Design review of the part built by this model. Coordinates are the model's own, in mm. Face numbers are marked on the shaded views. Give positions to 0.01 mm unless a question says otherwise; leave off trailing zeros. Write each loop counter-clockwise with the first axis right and the second up, starting at its lowest first coordinate (ties: lowest second). Pieces come first, ordered by that corner, then holes. Notation, with made-up numbers: M -28.5,66.25 L -24.5,66.25 A13 ccw -24.5,91.25 Z; hole C 60.25,37 d1. An arc over 180 degrees is marked long. Answer in a Markdown table with one row per item.
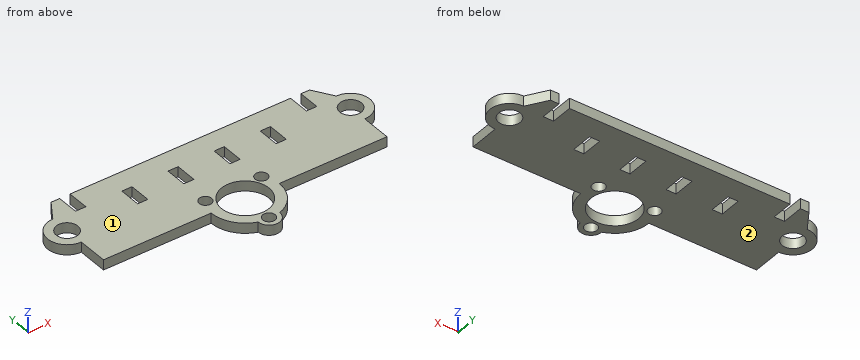
```python
from build123d import *

# Parameters (mm, degrees)
SKETCH2_R           = 7
SKETCH2_R_2         = 3.175
SKETCH2_R_3         = 1.8161
BOSS_EXTRUDE1_DEPTH = 2.9972
SKETCH3_W           = 2.9972
SKETCH3_H           = 6.35
CUT_EXTRUDE1_DEPTH  = 55.254506352


with BuildPart() as part:
    # Sketch2 → Boss-Extrude1 (new body)
    with BuildSketch(Plane.XY):
        with BuildLine():
            Line((-35.56, 26.035), (-38.1, 26.035))
            Line((-38.1, 26.035), (-41.790231571, 20.32))
            ThreePointArc((-41.790231571, 20.32), (-47.505231571, 14.605), (-41.790231571, 8.89))
            Line((-41.790231571, 8.89), (-41.790231571, 0))
            Line((-41.790231571, 0), (-10.040231571, 0))
            ThreePointArc((-10.040231571, 0), (-8.145059399, -5.87062666), (-3.175, -9.525))
            ThreePointArc((-3.175, -9.525), (0, -12.7), (3.175, -9.525))
            ThreePointArc((3.175, -9.525), (8.145059399, -5.87062666), (10.040231571, 0))
            Line((10.040231571, 0), (41.790231571, 0))
            Line((41.790231571, 0), (41.790231571, 8.89))
            ThreePointArc((41.790231571, 8.89), (47.505231571, 14.605), (41.790231571, 20.32))
            Line((41.790231571, 20.32), (38.1, 26.035))
            Line((38.1, 26.035), (35.56, 26.035))
            Line((35.56, 26.035), (35.56, 19.685))
            Line((35.56, 19.685), (32.512, 19.685))
            Line((32.512, 19.685), (32.512, 26.035))
            Line((32.512, 26.035), (-32.512, 26.035))
            Line((-32.512, 26.035), (-32.512, 19.685))
            Line((-32.512, 19.685), (-35.56, 19.685))
            Line((-35.56, 19.685), (-35.56, 26.035))
        make_face()
        with Locations(Location((0, 0, 0), (0, 0, 180))):
            Circle(SKETCH2_R, mode=Mode.SUBTRACT)
        with Locations(Location((-41.790231571, 14.605, 0), (0, 0, 180))):
            Circle(SKETCH2_R_2, mode=Mode.SUBTRACT)
        with Locations(Location((-8.248891971, 4.7625, 0), (0, 0, 180))):
            Circle(SKETCH2_R_3, mode=Mode.SUBTRACT)
        with Locations(Location((0, -9.525, 0), (0, 0, 180))):
            Circle(SKETCH2_R_3, mode=Mode.SUBTRACT)
        with Locations(Location((41.790231571, 14.605, 0), (0, 0, 180))):
            Circle(SKETCH2_R_2, mode=Mode.SUBTRACT)
        with Locations(Location((8.248891971, 4.7625, 0), (0, 0, 180))):
            Circle(SKETCH2_R_3, mode=Mode.SUBTRACT)
    extrude(amount=BOSS_EXTRUDE1_DEPTH)

    # Sketch3 → Cut-Extrude1 (cut, through all)
    with BuildSketch(Plane(origin=(0, 0, 0), x_dir=(-1, 0, 0), z_dir=(0, 0, -1))):
        with Locations((-20.40636, 16.51)):
            Rectangle(SKETCH3_W, SKETCH3_H)
        with Locations((-6.80212, 16.51)):
            Rectangle(SKETCH3_W, SKETCH3_H)
        with Locations((6.80212, 16.51)):
            Rectangle(SKETCH3_W, SKETCH3_H)
        with Locations((20.40636, 16.51)):
            Rectangle(SKETCH3_W, SKETCH3_H)
    extrude(amount=-CUT_EXTRUDE1_DEPTH, mode=Mode.SUBTRACT)


solid = part.part
```
1) Add section A-A (x = 0). Write out the cut boundary in (y, z) (3 decimals), and give its area (3 significant figures).
Geometry says:
| item | result |
|---|---|
| outline | M -12.7,0 L -11.341,0 L -11.341,2.997 L -12.7,2.997 Z; M -7.709,0 L -7,0 L -7,2.997 L -7.709,2.997 Z; M 7,0 L 26.035,0 L 26.035,2.997 L 7,2.997 Z |
| area | 63.2 mm^2 |
2) The part is to be moulded in two halves that separate along Z. For the marked faces 1 and 2, say which applies: released by +Z, released by -Z, zero draft, split by the parting line, or undercut.
Geometry says:
| item | result |
|---|---|
| face 1 | released by +Z |
| face 2 | released by -Z |
3) Add section C-C (x = 40). Write out the cut boundary in (y, z), and give its area (3 significant figures).
Geometry says:
| item | result |
|---|---|
| outline | M 0,0 L 11.98,0 L 11.98,3 L 0,3 Z; M 17.23,0 L 23.09,0 L 23.09,3 L 17.23,3 Z |
| area | 53.5 mm^2 |
4) To check wall thickness, follow probe 1 along Y at (x, z) = (0, 1.1) (3 decimals); probe 2 along X at (y, z) = (21, 0.15); probe 3 along X at (y, z) = (13, 0.9). State the ranges of each line that lie inside material, in increasing order. Write a range as [from, to].
Geometry says:
| item | result |
|---|---|
| probe 1 | [-12.7, -11.341], [-7.709, -7], [7, 26.035] |
| probe 2 | [-41.35, -35.56], [-32.51, 32.51], [35.56, 41.35] |
| probe 3 | [-47.28, -44.53], [-39.05, 39.05], [44.53, 47.28] |
5) Add section D-D (z = 1.3). Count the separate pieces of the cut face and the enclosed holes in it, and give its area (3 significant figures).
Geometry says:
| item | result |
|---|---|
| separate pieces | 1 |
| enclosed holes | 10 |
| area | 2,070 mm^2 |
6) Add section B-B (y = -2.5). Write out the cut boundary in (x, z), and give its area (3 significant figures).
Geometry says:
| item | result |
|---|---|
| outline | M -9.72,0 L -6.54,0 L -6.54,3 L -9.72,3 Z; M 6.54,0 L 9.72,0 L 9.72,3 L 6.54,3 Z |
| area | 19.1 mm^2 |
7) Insertion check: P1, Ø6, axis at x = -8.25, y = 4.76, coming from the -Z side; P2, Ø0.9, axis at y = 15.5, z = 2, coming from the +X side; P3, Ø1.5, axis at y = 17.5, z = 2, coming from the +X side; P4, Ø1, axis at y = 15.5, z = 2, coming from the -X side. Each pin has a flat end and moves straight along its axis. Give the tip position at first contact, or say it passes through.
Geometry says:
| item | result |
|---|---|
| P1 | z = 0 |
| P2 | x = 47.49 |
| P3 | x = 47.09 |
| P4 | x = -47.49 |
